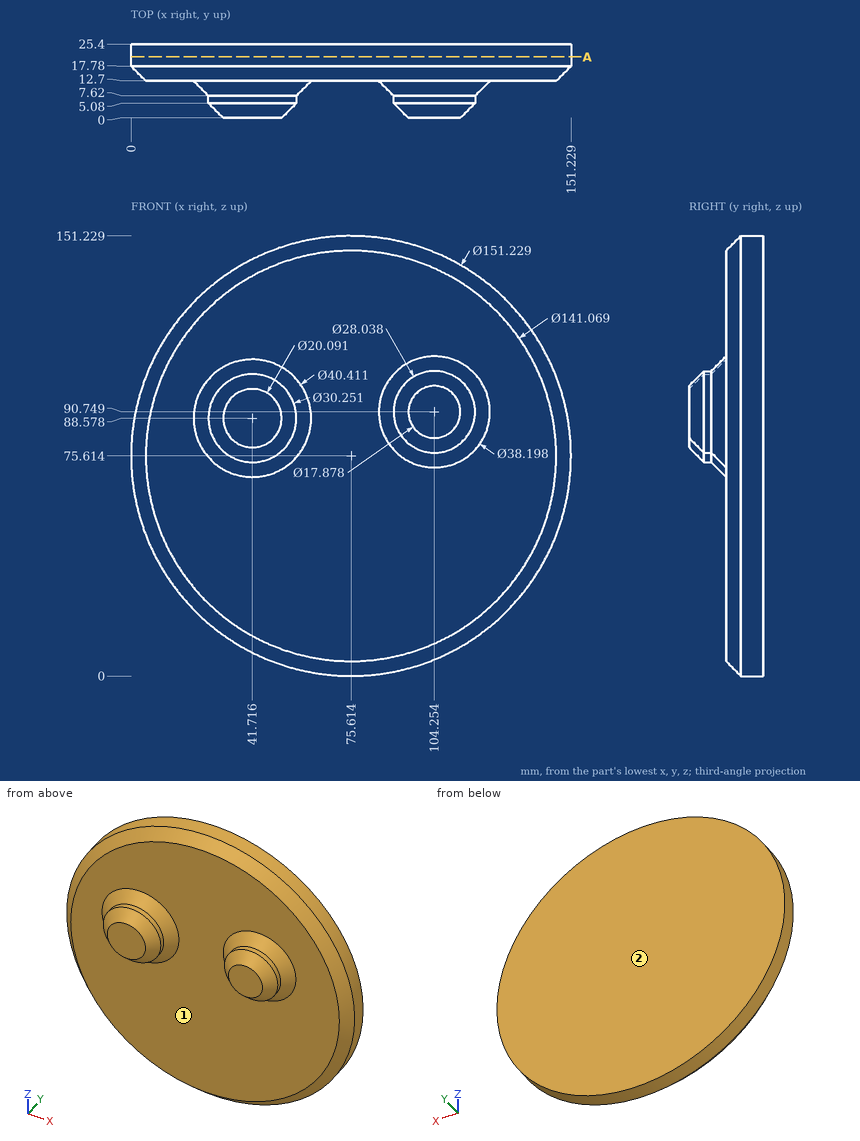
Print and shaded views of the part. All mm, measured from the part's lowest x, y and z. A direction names the side the tool comes from. Give positions to 0.01 mm unless a question says otherwise; leave off trailing zeros. Write each loop counter-clockwise with the first axis right and the second up, starting at its lowest first coordinate (ties: lowest second). Pieces come first, ordered by that corner, then holes. Notation, with made-up numbers: M -6,48 L 10,48 A30 ccw 10,85 Z; hole C 44.25,5.25 d3. An arc over 180 degrees is marked long. Use a Markdown table: item, result.
1) Tool access for the marked faces 1 and 2: list every direction of +Z, -Z, +X, -X, +Y, -Y with a clear straight run to the whole face (end or side of a thin tool).
Responses:
| item | result |
|---|---|
| face 1 | -Y |
| face 2 | +Z, -Z, +X, -X, +Y |
2) Drill centre lines: line 1 (Y direction, x = 101, z = 21); line 2 (Z direction, x = 17.5, y = 24.25) (1 decimal); line 3 (X direction, y = 21.75, z = 73) (1 decimal). Where is each one in solid material? Low to high. Write a range as from..to.
Responses:
| item | result |
|---|---|
| line 1 | y = 12.7..25.4 |
| line 2 | z = 27.2..124 |
| line 3 | x = 0..151.2 |
3) Pin check, flat tips, straight feed: pin 1 (1.5 mm diameter, centred on y = 13.5, z = 103.5, fed in from +X) (1 decimal); pin 2 (12 mm diameter, centred on y = 19, z = 63, fed in from +X); pin 3 (8 mm diameter, centred on y = 15, z = 110.5, fed in from +X). Stop position of each tip, or through.
Responses:
| item | result |
|---|---|
| pin 1 | stops at x = 142.1 |
| pin 2 | stops at x = 150.94 |
| pin 3 | stops at x = 144.12 |
4) Cut at A-A (y = 21). List the corners of the cut face in (x, z) (1 decimal).
Responses:
| item | result |
|---|---|
| outline | C 75.6,75.6 d151.2 |
